For this review, take the finished solid that the model builds, in its own axes (mm). Coordinates: 2 decimals unless noted, no trailing zeros. Loops run counter-clockwise (first coordinate to the right, second up) from the corner with the lowest first, then second, coordinate; pieces in that order, holes last. Notation, with made-up numbers: (36, -17) -> (95, -17) arc R10 ccw to (95, -3) -> close; hole circle Ø8 at (-13.75, -15). An arc over 180 degrees is marked (long way). Use a Markdown table: item, result.
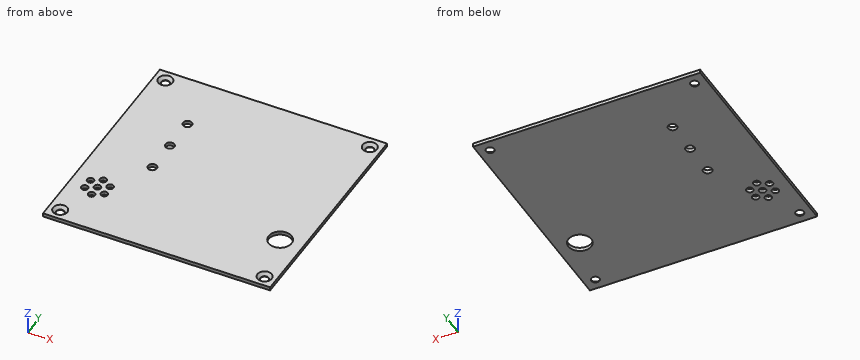
from build123d import *

# Parameters (mm, degrees)
ESQUISSE1_W                                 = 100
ESQUISSE1_H                                 = 100
BOSS_EXTRU_1_DEPTH                          = 1.6
FRAISAGE_POUR_VIS_T_TE_FRAIS_E_M31_AT_COUNT = 2
FRAISAGE_POUR_VIS_T_TE_FRAIS_E_M31_AT_PITCH = 90
FRAISAGE_POUR_VIS_T_TE_FRAIS_E_M31_2_COUNT  = 2
FRAISAGE_POUR_VIS_T_TE_FRAIS_E_M31_2_PITCH  = 127.279220614
FRAISAGE_POUR_VIS_T_TE_FRAIS_E_M31_3_COUNT  = 2
FRAISAGE_POUR_VIS_T_TE_FRAIS_E_M31_3_PITCH  = 90
ESQUISSE4_R                                 = 5.05
ESQUISSE4_R_2                               = 1.5
ESQUISSE4_R_3                               = 1.95
ENL_V_MAT_EXTRU_1_DEPTH                     = 2.6


with BuildPart() as part:
    # Esquisse1 → Boss.-Extru.1 (new body)
    with BuildSketch(Plane.XY):
        with Locations((50, 50)):
            Rectangle(ESQUISSE1_W, ESQUISSE1_H)
    extrude(amount=BOSS_EXTRU_1_DEPTH)

    # Esquisse3 → Fraisage pour vis à tête fraisée M31 (revolve, cut)
    with BuildSketch(Plane(origin=(5, 95, 1.6), x_dir=(0, -1, 0), z_dir=(1, 0, 0))):
        Polygon((0, 0), (0, 1.6), (1.8, 1.6), (1.8, 1.35), (3.15, 0), align=None)
    fraisage_pour_vis_t_te_frais_e_m31 = revolve(axis=Axis((5, 95, 7.95), (0, 0, -1)), mode=Mode.SUBTRACT)

    # Fraisage pour vis à tête fraisée M31 at: Fraisage pour vis à tête fraisée M31 ×2
    with Locations(*[(i * FRAISAGE_POUR_VIS_T_TE_FRAIS_E_M31_AT_PITCH, 0, 0) for i in range(1, FRAISAGE_POUR_VIS_T_TE_FRAIS_E_M31_AT_COUNT)]):
        add(fraisage_pour_vis_t_te_frais_e_m31, mode=Mode.SUBTRACT)

    # Fraisage pour vis _ t_te frais_e M31 2: Fraisage pour vis à tête fraisée M31 ×2
    with Locations(*[Vector(0.707106781, -0.707106781, 0) * (i * FRAISAGE_POUR_VIS_T_TE_FRAIS_E_M31_2_PITCH) for i in range(1, FRAISAGE_POUR_VIS_T_TE_FRAIS_E_M31_2_COUNT)]):
        add(fraisage_pour_vis_t_te_frais_e_m31, mode=Mode.SUBTRACT)

    # Fraisage pour vis _ t_te frais_e M31 3: Fraisage pour vis à tête fraisée M31 ×2
    with Locations(*[(0, -i * FRAISAGE_POUR_VIS_T_TE_FRAIS_E_M31_3_PITCH, 0) for i in range(1, FRAISAGE_POUR_VIS_T_TE_FRAIS_E_M31_3_COUNT)]):
        add(fraisage_pour_vis_t_te_frais_e_m31, mode=Mode.SUBTRACT)

    # Esquisse4 → Enlèv. mat.-Extru.1 (cut, through all)
    with BuildSketch(Plane.XY.offset(1.6)):
        with Locations((90, 28)):
            Circle(ESQUISSE4_R)
        with Locations((11.557, 24.13)):
            Circle(ESQUISSE4_R_2)
        with Locations((11.557, 29.13)):
            Circle(ESQUISSE4_R_2)
        with Locations((15.887127019, 26.63)):
            Circle(ESQUISSE4_R_2)
        with Locations((15.887127019, 21.63)):
            Circle(ESQUISSE4_R_2)
        with Locations((11.557, 19.13)):
            Circle(ESQUISSE4_R_2)
        with Locations((7.226872981, 21.63)):
            Circle(ESQUISSE4_R_2)
        with Locations((7.226872981, 26.63)):
            Circle(ESQUISSE4_R_2)
        with Locations((25, 75)):
            Circle(ESQUISSE4_R_3)
        with Locations((25, 60)):
            Circle(ESQUISSE4_R_3)
        with Locations((25, 45)):
            Circle(ESQUISSE4_R_3)
    extrude(amount=-ENL_V_MAT_EXTRU_1_DEPTH, mode=Mode.SUBTRACT)


solid = part.part
(1) Take a section at D-D on x = 87. Write out the cut boundary in (y, z).
Found:
| item | result |
|---|---|
| outline | (0, 0) -> (23.94, 0) -> (23.94, 1.6) -> (0, 1.6) -> close; (32.06, 0) -> (100, 0) -> (100, 1.6) -> (32.06, 1.6) -> close |
(2) For line 1 along Y through (x, z) = (5, 0.1); line 2 along Y through (x, z) = (90, 0.5); line 3 along Y through (x, z) = (15, 1.1), list the stretches that pass through material, from the lowest coordinate up.
Found:
| item | result |
|---|---|
| line 1 | y = 0 to 3.2, 6.8 to 93.2, 96.8 to 100 |
| line 2 | y = 0 to 22.95, 33.05 to 100 |
| line 3 | y = 0 to 20.42, 22.84 to 25.42, 27.84 to 100 |
(3) Take a section at B-B on z = 0.5. State how many separate pieces and enclosed holes the cut face has, plus the area to 3 significant figures.
Found:
| item | result |
|---|---|
| separate pieces | 1 |
| enclosed holes | 15 |
| area | 9,780 mm^2 |
(4) For pin 1 Ø3 at (x, y) = (5, 95) entering from +Z, flat-tipped, find the tip position at first contact; note if it passes through.
Found:
| item | result |
|---|---|
| pin 1 | passes through |
(5) Take a section at C-C on y = 95. Write out the cut boundary in (x, z), plus the area to 3 significant figures.
Found:
| item | result |
|---|---|
| outline | (0, 0) -> (3.2, 0) -> (3.2, 0.25) -> (1.85, 1.6) -> (0, 1.6) -> close; (6.8, 0) -> (93.2, 0) -> (93.2, 0.25) -> (91.85, 1.6) -> (8.15, 1.6) -> (6.8, 0.25) -> close; (96.8, 0) -> (100, 0) -> (100, 1.6) -> (98.15, 1.6) -> (96.8, 0.25) -> close |
| area | 145 mm^2 |
(6) Take a section at A-A on y = 60. Write out the cut boundary in (x, z), plus the area to 3 significant figures.
Found:
| item | result |
|---|---|
| outline | (0, 0) -> (23.05, 0) -> (23.05, 1.6) -> (0, 1.6) -> close; (26.95, 0) -> (100, 0) -> (100, 1.6) -> (26.95, 1.6) -> close |
| area | 154 mm^2 |
